Verification items for the finished model (mm, model axes). Round coordinates to 2 decimals unless told otherwise and drop trailing zeros. Order: outer loops, then holes, each group sorted by start corner. A loop starts at its lowest first (then second) coordinate and runs counter-clockwise, first axis right, second up. Notation, with made-up numbers: M 34.5,0 L 42.5,0 A12 cw 42.5,19 Z; hole C 46,-19.75 d6. An arc over 180 degrees is marked long. Answer as a JSON object with one key per item and string values. Group by question number.
```python
from build123d import *

# Parameters (mm, degrees)
SKETCH1_R           = 72.3
SKETCH1_R_2         = 1.4
BOSS_EXTRUDE1_DEPTH = 4
CHAMFER1_SIZE       = 2


# Read off the part's stored shape, not the designer's step: CirPattern4
with BuildPart() as part:
    # Sketch1 → Boss-Extrude1 (new body)
    with BuildSketch(Plane(origin=(0, 0, 0), x_dir=(-1, 0, 0), z_dir=(0, 1, 0))):
        with Locations(Location((28.500199727, 0, 0), (0, 0, 90))):
            Circle(SKETCH1_R)
        with Locations(Location((28.500199727, 68, 0), (0, 0, 90))):
            Circle(SKETCH1_R_2, mode=Mode.SUBTRACT)
    extrude(amount=BOSS_EXTRUDE1_DEPTH)

    # Chamfer1
    chamfer1_edges = [part.edges().sort_by_distance(p)[0] for p in [
        (-28.500199727, 4, 66.6),
    ]]
    chamfer(chamfer1_edges, length=CHAMFER1_SIZE)

    # CirPattern4 outline → CirPattern4 (revolve, cut)
    with BuildSketch(Plane(origin=(-93.172042835, 0, 21.013155617), x_dir=(1, 0, 0), z_dir=(0, 0, 1))):
        Polygon((3.4, 4), (0, 4), (0, 0), (1.4, 0), (1.4, 2), align=None)
    revolve(axis=Axis((-93.172042835, 0, 21.013155617), (0, 1, 0)), mode=Mode.SUBTRACT)

    # CirPattern4 2 outline → CirPattern4 2 (revolve, cut)
    with BuildSketch(Plane(origin=(-68.469596883, 0, -55.013155617), x_dir=(1, 0, 0), z_dir=(0, 0, 1))):
        Polygon((3.4, 4), (0, 4), (0, 0), (1.4, 0), (1.4, 2), align=None)
    revolve(axis=Axis((-68.469596883, 0, -55.013155617), (0, 1, 0)), mode=Mode.SUBTRACT)

    # CirPattern4 3 outline → CirPattern4 3 (revolve, cut)
    with BuildSketch(Plane(origin=(11.469197429, 0, -55.013155617), x_dir=(1, 0, 0), z_dir=(0, 0, 1))):
        Polygon((3.4, 4), (0, 4), (0, 0), (1.4, 0), (1.4, 2), align=None)
    revolve(axis=Axis((11.469197429, 0, -55.013155617), (0, 1, 0)), mode=Mode.SUBTRACT)

    # CirPattern4 4 outline → CirPattern4 4 (revolve, cut)
    with BuildSketch(Plane(origin=(36.171643381, 0, 21.013155617), x_dir=(1, 0, 0), z_dir=(0, 0, 1))):
        Polygon((3.4, 4), (0, 4), (0, 0), (1.4, 0), (1.4, 2), align=None)
    revolve(axis=Axis((36.171643381, 0, 21.013155617), (0, 1, 0)), mode=Mode.SUBTRACT)


solid = part.part
```
Q1. Cross-section at B-B, the plane z = -31.5. Record the cut outline in (x, y).
Q2. Gauge pin test, flat ends, axial feed: pin 1 Ø1.5 at (x, y) = (-30.5, 3) entering from +Z; pin 2 Ø1 at (y, z) = (3, -23) entering from -X; pin 3 Ø3 at (x, z) = (-93.17, 21.01) entering from +Y. Record the tip position at first contact, or that the pin passes through.
Q3. Release check for a two-part mould opening along X. For faces 1 (the face through (-27, 4, -1)), 2 (the face through (-72.494, 1.972, -57.375)), 3 (the face through (11.14, 2.13, -53.52)), 4 (the face through (-94.382, 2.125, 21.941)) record: released by +X, released by -X, zero draft, split by the parting line, or undercut.
Q4. Cross-section at C-C, the plane x = -43.5. Record the cut outline in (y, z).
Q5. Thickness scan on line 1 (X direction, y = 0.9, z = 21.5); line 2 (X direction, y = 2.55, z = -1.5); line 3 (Z direction, x = 11.5, y = 2.1). Record the ranges inside material, lowest first. Write a range as from..to.
Q6. Cross-section at A-A, the plane y = 0.85. Record the cut outline in (x, z), then the cut area to 3 significant figures.
Conclusion:
{
 "1": {"outline": "M -93.58,0 L 36.58,0 L 36.58,4 L -93.58,4 Z"},
 "2": {"pin 1": "z = 72.29", "pin 2": "x = -97.21", "pin 3": "y = 2.1"},
 "3": {"face 1": "zero draft", "face 2": "split by the parting line", "face 3": "undercut", "face 4": "undercut"},
 "4": {"outline": "M 0,-70.73 L 4,-70.73 L 4,70.73 L 0,70.73 Z"},
 "5": {"line 1": "-97.53..-94.48, -91.86..34.86, 37.48..40.53", "line 2": "-100.78..43.78", "line 3": "-60.23..-56.51, -53.51..60.23"},
 "6": {"outline": "C -28.5,0 d144.6; hole C -93.17,21.01 d2.8; hole C -68.47,-55.01 d2.8; hole C -28.5,68 d2.8; hole C 11.47,-55.01 d2.8; hole C 36.17,21.01 d2.8", "area": "16,400 mm2"}
}
